Source: CAD feature listing. Evaluate the final solid. Frame: model axes, mm. Face numbers are marked on the shaded views. A direction names the side the tool comes from. Coordinates: 2 decimals unless noted, no trailing zeros. Order: outer loops, then holes, each group sorted by start corner. A loop starts at its lowest first (then second) coordinate and runs counter-clockwise, first axis right, second up.
```python
from build123d import *
from build123d.topology import SkipClean

# Parameters (mm, degrees)
EXTRUDE_1_DEPTH     = 6
SKETCH_2_R          = 15.011106999
SKETCH_2_R_2        = 14.25
CUT_EXTRUDE_1_DEPTH = 21.744477177
EXTRUDE_START       = -1.5
SKETCH_4_R          = 14.25
EXTRUDE_3_DEPTH     = 1.5
SKETCH_5_R          = 9.2
CUT_EXTRUDE_2_DEPTH = 22.026768653
CHAMFER_1_SIZE      = 1


with BuildPart() as part:
    # Sketch 1 → Extrude 1 (new body)
    with BuildSketch(Plane.XY):
        Polygon((0, 15.011106999), (-13, 7.505553499), (-13, -7.505553499), (0, -15.011106999), (13, -7.505553499), (13, 7.505553499), align=None)
    extrude(amount=EXTRUDE_1_DEPTH)

    # Sketch 2 → Cut-Extrude 1 (cut, through all)
    with BuildSketch(Plane.XY.offset(6)):
        Circle(SKETCH_2_R)
        Circle(SKETCH_2_R_2, mode=Mode.SUBTRACT)
    extrude(amount=-CUT_EXTRUDE_1_DEPTH, mode=Mode.SUBTRACT)

    # Sketch 4 → Extrude 3 (add)
    with SkipClean():  # the faces are left unmerged after this step: merging them gives an invalid solid
        with BuildSketch(Plane(origin=(0, 0, 0), x_dir=(-1, 0, 0), z_dir=(0, 0, -1)).offset(EXTRUDE_START)):
            with Locations(Location((0, 0, 0), (0, 0, 155.822455166))):
                Circle(SKETCH_4_R)
        extrude(amount=EXTRUDE_3_DEPTH)
    add(part.part.scale(1), mode=Mode.REPLACE)  # the faces are merged on a copy

    # Sketch 5 → Cut-Extrude 2 (cut, through all)
    with BuildSketch(Plane.XY.offset(6)):
        Circle(SKETCH_5_R)
    extrude(amount=-CUT_EXTRUDE_2_DEPTH, mode=Mode.SUBTRACT)

    # Chamfer 1
    chamfer_1_edges = [part.edges().sort_by_distance(p)[0] for p in [
        (-9.2, 0, 0),
        (-9.2, 0, 6),
    ]]
    chamfer(chamfer_1_edges, length=CHAMFER_1_SIZE)


solid = part.part
```
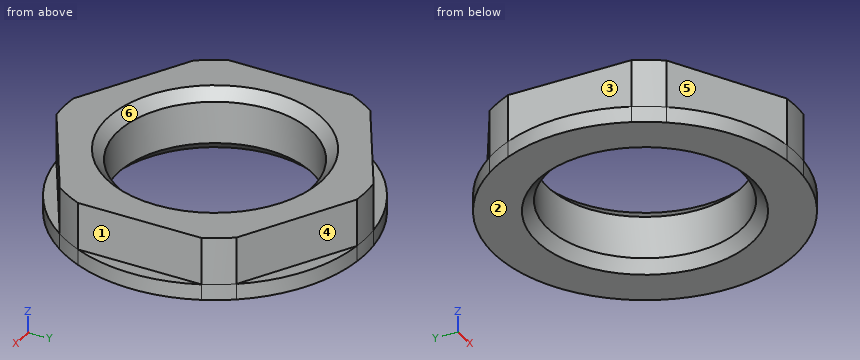
Q1. Pin query (flat end, axial travel): P1, Ø2, axis at x = -2, y = 8, coming from the +Z side; P2, Ø1.8, axis at x = 6, y = 12, coming from the +Z side; P3, Ø2, axis at y = -4, z = 4.5, coming from the +X side; P4, Ø2, axis at y = -11, z = 4.5, coming from the -X side. Return the tip coordinate at first contact, or that it passes through.
Solutions:
P1: stops at z = 5.05
P2: stops at z = 6
P3: stops at x = 13
P4: stops at x = -8.68
Q2. Pull-direction query (X, two-part tool) for the marked faces 4, 5 and 6; classes: pulls with the +X half, pulls with the -X half, needs draft (parallel to the pull), parting line crosses it, or undercut.
Solutions:
face 4: pulls with the +X half
face 5: pulls with the -X half
face 6: undercut
Q3. Section query C-C on z = 4.65. Output: boundary loops of the cut face in (x, y).
Solutions:
outline: (-13, -5.84) arc R14.25 ccw to (-11.55, -8.34) - (-1.45, -14.18) arc R14.25 ccw to (1.45, -14.18) - (11.55, -8.34) arc R14.25 ccw to (13, -5.84) - (13, 5.84) arc R14.25 ccw to (11.55, 8.34) - (1.45, 14.18) arc R14.25 ccw to (-1.45, 14.18) - (-11.55, 8.34) arc R14.25 ccw to (-13, 5.84) - close; hole circle Ø18.4 at (0, 0)
Q4. Section query D-D on y = 12.5. Output: boundary loops of the cut face in (x, z).
Solutions:
outline: (-6.84, 0) - (6.84, 0) - (6.84, 1.5) - (4.35, 1.5) - (4.35, 6) - (-4.35, 6) - (-4.35, 1.5) - (-6.84, 1.5) - close
Q5. Set-up query: the marked faces 1, 2 and 3. Return all of +Z, -Z, +X, -X, +Y, -Y with unobstructed straight access to the full face (end or side cutting, diameter ignored); none if empty.
Solutions:
face 1: +Z, +X, +Y, -Y
face 2: -Z, +X, -X, +Y, -Y
face 3: +Z, -X, +Y, -Y
Q6. Section query B-B on y = 0. Output: boundary loops of the cut face in (x, z).
Solutions:
outline: (-14.25, 0) - (-10.2, 0) - (-9.2, 1) - (-9.2, 5) - (-10.2, 6) - (-13, 6) - (-13, 1.5) - (-14.25, 1.5) - close; (9.2, 1) - (10.2, 0) - (14.25, 0) - (14.25, 1.5) - (13, 1.5) - (13, 6) - (10.2, 6) - (9.2, 5) - close
Q7. Section query A-A on x = 0. Output: boundary loops of the cut face in (y, z), plus the area to 3 significant figures.
Solutions:
outline: (-14.25, 0) - (-10.2, 0) - (-9.2, 1) - (-9.2, 5) - (-10.2, 6) - (-14.25, 6) - close; (9.2, 1) - (10.2, 0) - (14.25, 0) - (14.25, 6) - (10.2, 6) - (9.2, 5) - close
area: 58.6 mm2
Q8. Material intervals for line 1 along Y through (x, z) = (0, 3.9); line 2 along Y through (x, z) = (7.5, 3.9); line 3 along Z through (x, y) = (7, 12), sorted ascending.
Solutions:
line 1: y = -14.25 to -9.2, 9.2 to 14.25
line 2: y = -10.68 to -5.33, 5.33 to 10.68
line 3: z = 0 to 1.5
